Model file for the job. Use its own axes, mm. A direction names the side the tool comes from. Give positions to 0.01 mm unless a question says otherwise; leave off trailing zeros. Order: outer loops, then holes, each group sorted by start corner. A loop starts at its lowest first (then second) coordinate and runs counter-clockwise, first axis right, second up. Notation, with made-up numbers: (8.25, -28) -> (21.25, -28) arc R22 ccw to (21.25, -4) -> close; hole circle Ø3 at (15.25, 12.25). An arc over 180 degrees is marked (long way). Use CSV: the item, a comma, the result in double quotes. Start each with the question number.
1. Cut at C-C on x = -78.5. List the corners of the cut face in (y, z), then the cut area to 3 significant figures.
2. Wall check: line 1 (Y direction, x = 6, z = 121); line 2 (Y direction, x = -20, z = 29); line 3 (Z direction, x = -64.5, y = 38). Give the ranges that are in metal, low to high. Write a range as from..to.
3. Drop flat-ended pins along their axis: pin 1 (3 mm diameter, centred on x = -74, z = 74.5, fed in from +Y); pin 2 (15.5 mm diameter, centred on x = -29, z = 49, fed in from -Y); pin 3 (5.5 mm diameter, centred on x = -32.5, y = -120, fed in from -Z). Give the stop position or say it passes through.
4. 3-axis set-ups, long thin cutter, end or side, ignore diameter. For faces 1 (the flat face through (-23, -120, 103.9)), 2 (the flat face through (-48.658, -112, 129)), 3 (the flat face through (-23, -111.072, 121)): which of +Z, -Z, +X, -X, +Y, -Y reach the whole face in a straight line?
5. Cut at A-A on z = 121. List the corners of the cut face in (x, y), then the cut area to 3 significant figures.
6. Pull direction X, two halves, no side cores. Call faces 4 (the flat face through (-22, -50, 71)), 5 (the flat face through (-24, 1, 25)), 6 (the cylindrical face through (-113.642, 1.429, 70.992)), 7 (the flat face through (-30, -53, 144)): released by +X, released by -X, zero draft, split by the parting line, or undercut.
7. Cut at D-D on y = -72. List the corners of the cut face in (x, z), then the cut area to 3 significant figures.
8. Cut at B-B on z = 96.5. List the corners of the cut face in (x, y).
```python
from build123d import *

# Parameters (mm, degrees)
F1_DEPTH = 144
F2_W     = 52.2887532134
F2_H     = 46.0724334717
F3_DEPTH = 6.9
F2_H_2   = 17.8235247731
F4_DEPTH = 40.1
F5_DEPTH = 25


with BuildPart() as f1:
    # F0 (on Top) → F1 (new body)
    with BuildSketch(Plane.XY):
        with BuildLine():
            ThreePointArc((-22.5135510555, -59.5102644243), (-35.3006672315, -63.6127628215), (-48.6579276621, -65))
            Line((-48.6579276621, -65), (3.6308255512, -65))
            ThreePointArc((3.6308255512, -65), (-9.7264348794, -63.6127628215), (-22.5135510555, -59.5102644243))
        make_face()
        with BuildLine():
            ThreePointArc((-22.5135510555, 59.5102644243), (-35.3006672315, 63.6127628215), (-48.6579276621, 65))
            ThreePointArc((-48.6579276621, 65), (-113.6579276621, 0), (-48.6579276621, -65))
            ThreePointArc((-48.6579276621, -65), (-35.3006672315, -63.6127628215), (-22.5135510555, -59.5102644243))
            ThreePointArc((-22.5135510555, -59.5102644243), (-30.5403925409, -55.2931085589), (-37.9022937634, -50))
            Line((-37.9022937634, -50), (-48.6579276621, -50))
            ThreePointArc((-48.6579276621, -50), (-98.6579276621, 0), (-48.6579276621, 50))
            Line((-48.6579276621, 50), (-37.9022937634, 50))
            ThreePointArc((-37.9022937634, 50), (-30.5403925409, 55.2931085589), (-22.5135510555, 59.5102644243))
        make_face()
        with BuildLine():
            Line((3.6308255512, 65), (-48.6579276621, 65))
            ThreePointArc((-48.6579276621, 65), (-35.3006672315, 63.6127628215), (-22.5135510555, 59.5102644243))
            ThreePointArc((-22.5135510555, 59.5102644243), (-9.7264348794, 63.6127628215), (3.6308255512, 65))
        make_face()
        with BuildLine():
            ThreePointArc((3.6308255512, 65), (-9.7264348794, 63.6127628215), (-22.5135510555, 59.5102644243))
            ThreePointArc((-22.5135510555, 59.5102644243), (-14.48670957, 55.2931085589), (-7.1248083475, 50))
            Line((-7.1248083475, 50), (3.6308255512, 50))
            ThreePointArc((3.6308255512, 50), (38.9861646106, 35.3553390593), (53.6308255512, 0))
            ThreePointArc((53.6308255512, 0), (38.9861646106, -35.3553390593), (3.6308255512, -50))
            Line((3.6308255512, -50), (-7.1248083475, -50))
            ThreePointArc((-7.1248083475, -50), (-14.48670957, -55.2931085589), (-22.5135510555, -59.5102644243))
            ThreePointArc((-22.5135510555, -59.5102644243), (-9.7264348794, -63.6127628215), (3.6308255512, -65))
            ThreePointArc((3.6308255512, -65), (49.5927663284, -45.9619407771), (68.6308255512, 0))
            ThreePointArc((68.6308255512, 0), (49.5927663284, 45.9619407771), (3.6308255512, 65))
        make_face()
        with BuildLine():
            ThreePointArc((-7.1248083475, 50), (-14.48670957, 55.2931085589), (-22.5135510555, 59.5102644243))
            ThreePointArc((-22.5135510555, 59.5102644243), (-30.5403925409, 55.2931085589), (-37.9022937634, 50))
            Line((-37.9022937634, 50), (-7.1248083475, 50))
        make_face()
        with BuildLine():
            ThreePointArc((-37.9022937634, -50), (-30.5403925409, -55.2931085589), (-22.5135510555, -59.5102644243))
            ThreePointArc((-22.5135510555, -59.5102644243), (-14.48670957, -55.2931085589), (-7.1248083475, -50))
            Line((-7.1248083475, -50), (-37.9022937634, -50))
        make_face()
    extrude(amount=F1_DEPTH)

    # F2 (on face) → F3 (join)
    with BuildSketch(Plane.XY.offset(144)):
        with Locations((-22.5135510555, -88.0362167358)):
            Rectangle(F2_W, F2_H)
    extrude(amount=-F3_DEPTH)

    # F2 (on face) → F4 (join)
    with BuildSketch(Plane.XY.offset(144)):
        with Locations((-22.5135510555, -119.9841958582)):
            Rectangle(F2_W, F2_H_2)
    extrude(amount=-F4_DEPTH)

    # F0 (on Top) → F5 (join)
    with BuildSketch(Plane.XY):
        with BuildLine():
            ThreePointArc((-39.0084939829, -49.060049222), (-61.3691744488, 0), (-39.0084939829, 49.060049222))
            ThreePointArc((-39.0084939829, 49.060049222), (-43.810374728, 49.7644575028), (-48.6579276621, 50))
            ThreePointArc((-48.6579276621, 50), (-98.6579276621, 0), (-48.6579276621, -50))
            ThreePointArc((-48.6579276621, -50), (-43.810374728, -49.7644575028), (-39.0084939829, -49.060049222))
        make_face()
        with BuildLine():
            ThreePointArc((-22.5135510555, 42.620084137), (-30.473662451, 46.5760936396), (-39.0084939829, 49.060049222))
            ThreePointArc((-39.0084939829, 49.060049222), (-61.3691744488, 0), (-39.0084939829, -49.060049222))
            ThreePointArc((-39.0084939829, -49.060049222), (-30.473662451, -46.5760936396), (-22.5135510555, -42.620084137))
            ThreePointArc((-22.5135510555, -42.620084137), (-46.3691744488, 0), (-22.5135510555, 42.620084137))
        make_face()
        with BuildLine():
            ThreePointArc((1.3420723379, 0), (-5.0275550398, 24.4211094104), (-22.5135510555, 42.620084137))
            ThreePointArc((-22.5135510555, 42.620084137), (-46.3691744488, 0), (-22.5135510555, -42.620084137))
            ThreePointArc((-22.5135510555, -42.620084137), (-5.0275550398, -24.4211094104), (1.3420723379, 0))
        make_face()
        with BuildLine():
            ThreePointArc((16.3420723379, 0), (10.4883138487, 26.9577839435), (-6.018608128, 49.060049222))
            ThreePointArc((-6.018608128, 49.060049222), (-14.55343966, 46.5760936396), (-22.5135510555, 42.620084137))
            ThreePointArc((-22.5135510555, 42.620084137), (-5.0275550398, 24.4211094104), (1.3420723379, 0))
            ThreePointArc((1.3420723379, 0), (-5.0275550398, -24.4211094104), (-22.5135510555, -42.620084137))
            ThreePointArc((-22.5135510555, -42.620084137), (-14.55343966, -46.5760936396), (-6.018608128, -49.060049222))
            ThreePointArc((-6.018608128, -49.060049222), (10.4883138487, -26.9577839435), (16.3420723379, 0))
        make_face()
        with BuildLine():
            ThreePointArc((3.6308255512, 50), (-1.2167273829, 49.7644575028), (-6.018608128, 49.060049222))
            ThreePointArc((-6.018608128, 49.060049222), (10.4883138487, 26.9577839435), (16.3420723379, 0))
            ThreePointArc((16.3420723379, 0), (10.4883138487, -26.9577839435), (-6.018608128, -49.060049222))
            ThreePointArc((-6.018608128, -49.060049222), (-1.2167273829, -49.7644575028), (3.6308255512, -50))
            ThreePointArc((3.6308255512, -50), (38.9861646106, -35.3553390593), (53.6308255512, 0))
            ThreePointArc((53.6308255512, 0), (38.9861646106, 35.3553390593), (3.6308255512, 50))
        make_face()
    extrude(amount=F5_DEPTH)


solid = f1.part
```
Verdict:
1,outline,"(-57.74, 0) -> (57.74, 0) -> (57.74, 144) -> (40.12, 144) -> (40.12, 25) -> (-40.12, 25) -> (-40.12, 144) -> (-57.74, 144) -> close"
1,area,"7,080 mm^2"
2,line 1,"-64.96..-49.94, 49.94..64.96"
2,line 2,"-65..-50, 50..65"
2,line 3,"0..25"
3,pin 1,"y = 60.47"
3,pin 2,"y = -65"
3,pin 3,"z = 103.9"
4,face 1,"-Z, +X, -X, -Y"
4,face 2,"+Z, -Z, -X, -Y"
4,face 3,"-Z, +X, -X"
5,outline,"(-48.66, -128.9) -> (3.63, -128.9) -> (3.63, -111.07) -> (-48.66, -111.07) -> close; (-48.66, -65) -> (3.63, -65) arc R65 ccw to (3.63, 65) -> (-48.66, 65) arc R65 ccw to start; hole (-48.66, -50) -> (3.63, -50) arc R50 ccw to (3.63, 50) -> (-48.66, 50) arc R50 ccw to start"
5,area,"7,920 mm^2"
6,face 4,"undercut"
6,face 5,"undercut"
6,face 6,"released by -X"
6,face 7,"zero draft"
7,outline,"(-48.66, 137.1) -> (3.63, 137.1) -> (3.63, 144) -> (-48.66, 144) -> close"
7,area,"361 mm^2"
8,outline,"(-48.66, -65) -> (3.63, -65) arc R65 ccw to (3.63, 65) -> (-48.66, 65) arc R65 ccw to start; hole (-48.66, -50) -> (3.63, -50) arc R50 ccw to (3.63, 50) -> (-48.66, 50) arc R50 ccw to start"
